Source: three-view drawing plus pictorial views. Frame: mm from the lowest corner of the part. A direction names the side the tool comes from. Give positions to 0.01 mm unless a question says otherwise; leave off trailing zeros. Loops run counter-clockwise (first coordinate to the right, second up) from the corner with the lowest first, then second, coordinate; pieces in that order, holes last. Notation, with made-up numbers: (-14, 46.5) - (17, 46.5) arc R26 cw to (17, 82.5) - close; hole circle Ø2 at (74.25, 72.5). An arc over 180 degrees is marked (long way). Answer as a JSON object with one key per item and string values.
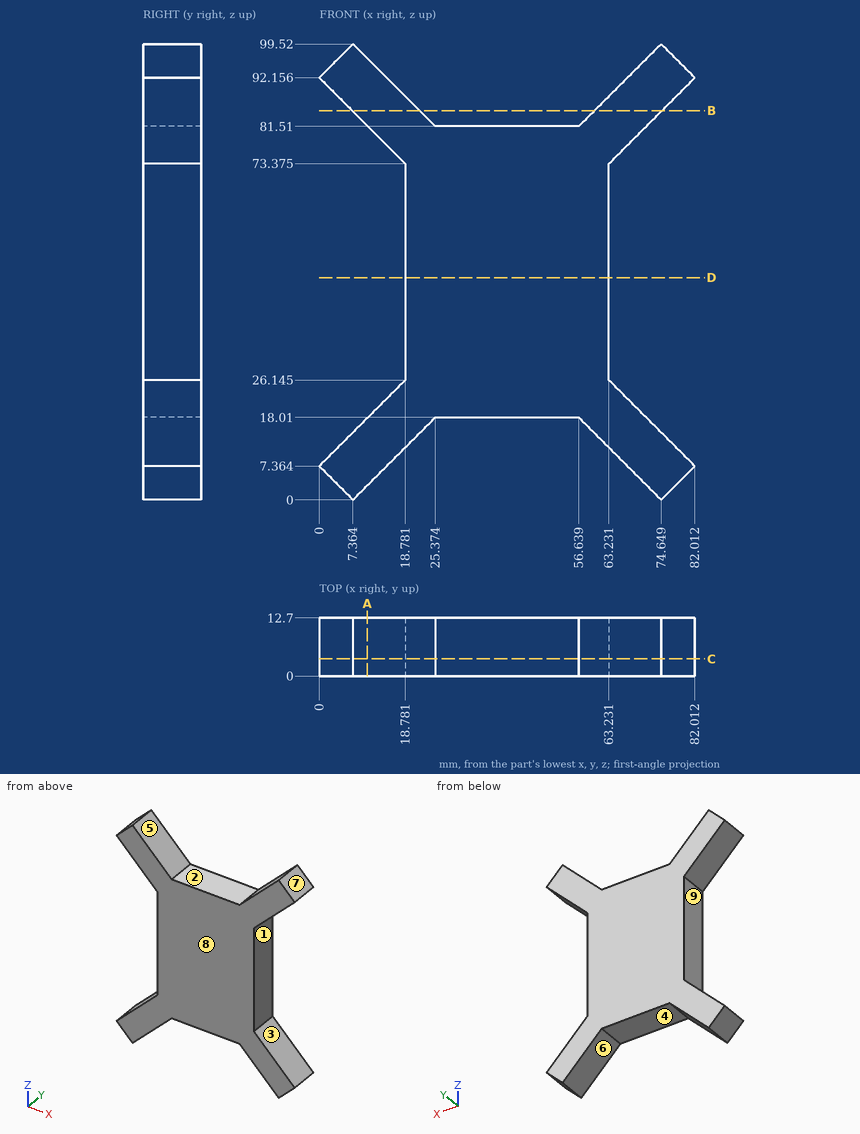
Item 1: Material intervals for line 1 (X direction, y = 11.5, z = 69.5); line 2 (X direction, y = 8.5, z = 90.5) (1 decimal); line 3 (Z direction, x = 39, y = 8.5), sorted ascending. Write a range as [from, to].
Geometry check:
{"line 1": "x = [18.78, 63.23]", "line 2": "x = [1.7, 16.4], [65.6, 80.4]", "line 3": "z = [18.01, 81.51]"}
Item 2: Mould query, pull axis Z, two halves, no side actions, for the marked faces 1, 2, 3 and 4. Classes: released by +Z, released by -Z, zero draft, split by the parting line, or undercut.
Geometry check:
{"face 1": "undercut", "face 2": "released by +Z", "face 3": "undercut", "face 4": "released by -Z"}
Item 3: Contact query for flat-ended pins moving along their axis: P1, Ø4, axis at x = 48.5, y = 7, coming from the -Z side; P2, Ø2, axis at y = 6.5, z = 83.5, coming from the -X side (1 decimal); P3, Ø3, axis at x = 51.5, y = 9, coming from the +Z side. Output: stop coordinate, or through.
Geometry check:
{"P1": "stops at z = 18.01", "P2": "stops at x = 7.7", "P3": "stops at z = 81.51"}
Item 4: Access query for the marked faces 5, 6, 7, 8 and 9. Directions: +Z, -Z, +X, -X, +Y, -Y. A direction counts if a zero-diameter tool reaches every point of the face in a straight line with its end or side. Return the directions, or none.
Geometry check:
{"face 5": "+Z, +Y, -Y", "face 6": "-Z, +Y, -Y", "face 7": "+Z, +X, +Y, -Y", "face 8": "+Z, -Z, +X, -X, -Y", "face 9": "-X, +Y, -Y"}
Item 5: Cut plane B-B (z = 85). Return loops of the section in (x, y).
Geometry check:
{"outline": "(7.16, 0) - (21.88, 0) - (21.88, 12.7) - (7.16, 12.7) - close; (60.13, 0) - (74.86, 0) - (74.86, 12.7) - (60.13, 12.7) - close"}
Item 6: Cut plane A-A (x = 10.5). Return loops of the section in (y, z), then the cut area to 3 significant figures.
Geometry check:
{"outline": "(0, 3.14) - (12.7, 3.14) - (12.7, 17.86) - (0, 17.86) - close; (0, 81.66) - (12.7, 81.66) - (12.7, 96.38) - (0, 96.38) - close", "area": "374 mm2"}
Item 7: Cut plane D-D (z = 48.5). Return loops of the section in (x, y).
Geometry check:
{"outline": "(18.78, 0) - (63.23, 0) - (63.23, 12.7) - (18.78, 12.7) - close"}
Item 8: Cut plane C-C (y = 3.75). Return loops of the section in (x, z) (1 decimal), then the cut area to 3 significant figures.
Geometry check:
{"outline": "(0, 7.4) - (7.4, 0) - (25.4, 18) - (56.6, 18) - (74.6, 0) - (82, 7.4) - (63.2, 26.1) - (63.2, 73.4) - (82, 92.2) - (74.6, 99.5) - (56.6, 81.5) - (25.4, 81.5) - (7.4, 99.5) - (0, 92.2) - (18.8, 73.4) - (18.8, 26.1) - close", "area": "3,800 mm2"}
